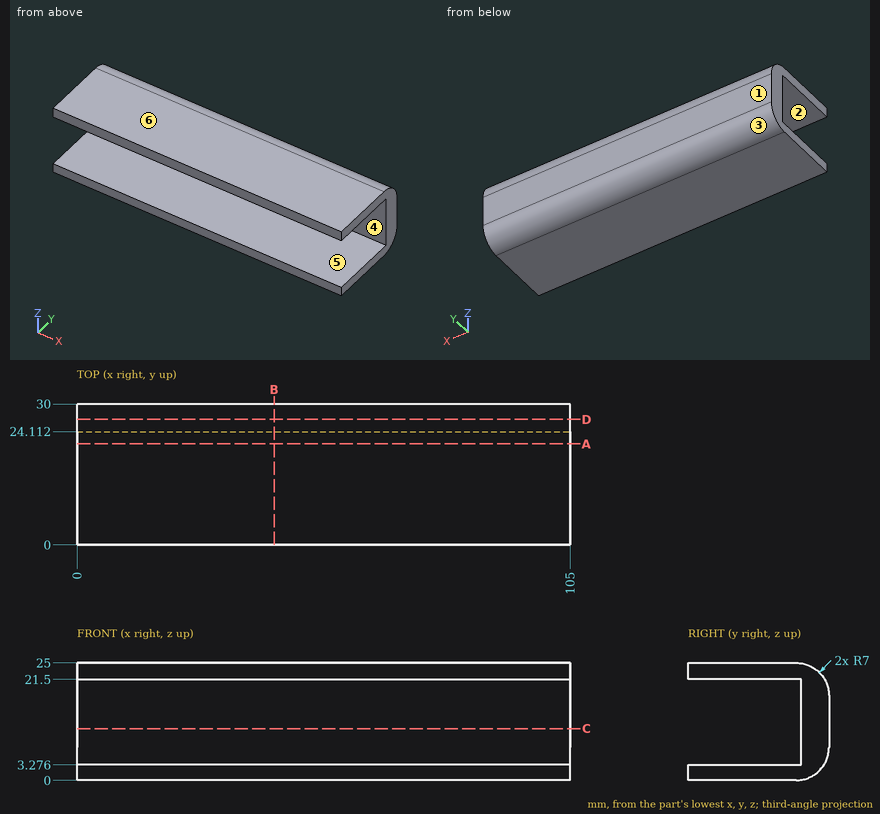
Could you check a few things on this drawing? It's one solid part, dimensions in mm from its lowest x, y, z. A direction names the side the tool comes from. Give positions to 0.01 mm unless a question says otherwise; leave off trailing zeros. Order: outer loops, then holes, each group sorted by start corner. A loop starts at its lowest first (then second) coordinate and runs counter-clockwise, first axis right, second up. Notation, with made-up numbers: (66, -2.75) - (97, -2.75) arc R14 cw to (97, 21.25) - close; hole circle Ø3 at (-18.5, 45). An arc over 180 degrees is marked (long way). Return JSON: item names as keys, results as strings. Group by question number.
Q1. Which directions (+Z, -Z, +X, -X, +Y, -Y) give clear straight access to the entire face, cutting with the end or side of a thin tool? Please do the marked faces 5 and 6.
Q2. Please list where these lines run through material, in increasing order: line 1 along Z through (x, y) = (53.5, 20); line 2 along Y through (x, z) = (37, 11.5); line 3 along Y through (x, z) = (83, 19). Write a range as [from, to].
Q3. Suppose I cut it at A-A, the plane y = 21.5. Please give me the cut outline in (x, z).
Q4. Suppose I cut it at B-B, the plane x = 42. Please give me the cut outline in (y, z).
Q5. Suppose I cut it at C-C, the plane z = 11. Please give me the cut outline in (x, y).
Q6. Will these pins go through, and if not, where does the flat tip stop? pin 1 Ø1 at (x, y) = (18.5, 25) entering from +Z; pin 2 Ø2 at (y, z) = (23, 17) entering from +X.
Q7. Thinking about a two-plate mould opening in Z: for the marked faces 1, 2, 3 and 4, which applies, pulls with the +Z half, pulls with the -Z half, needs draft (parallel to the pull), parting line crosses it, or undercut?
Q8. Suppose I cut it at D-D, the plane y = 26.75. Please give me the cut outline in (x, z).
Resolved:
{
 "1": {"face 5": "+X, -X, -Y", "face 6": "+Z, +X, -X, +Y, -Y"},
 "2": {"line 1": "z = [0, 3.28], [21.5, 25]", "line 2": "y = [24.11, 30]", "line 3": "y = [24.11, 29.93]"},
 "3": {"outline": "(0, 0) - (105, 0) - (105, 3.28) - (0, 3.28) - close; (0, 21.5) - (105, 21.5) - (105, 25) - (0, 25) - close"},
 "4": {"outline": "(0, 0) - (23, 0) arc R7 ccw to (30, 7) - (30, 18) arc R7 ccw to (23, 25) - (0, 25) - (0, 21.5) - (24.11, 21.5) - (24.11, 3.28) - (0, 3.28) - close"},
 "5": {"outline": "(0, 24.11) - (105, 24.11) - (105, 30) - (0, 30) - close"},
 "6": {"pin 1": "stops at z = 24.84", "pin 2": "passes through"},
 "7": {"face 1": "needs draft", "face 2": "undercut", "face 3": "pulls with the -Z half", "face 4": "undercut"},
 "8": {"outline": "(0, 1.09) - (105, 1.09) - (105, 23.91) - (0, 23.91) - close"}
}
